Here's how the part is built. I have some questions about the finished solid (model axes, mm). Face numbers are marked on the shaded views. A direction names the side the tool comes from. Coordinates: 2 decimals unless noted, no trailing zeros. Loops run counter-clockwise (first coordinate to the right, second up) from the corner with the lowest first, then second, coordinate; pieces in that order, holes last. Notation, with made-up numbers: (74, -17) -> (122, -17) arc R7 ccw to (122, -7) -> close; hole circle Ø4 at (70, 32.25). An arc over 180 degrees is marked (long way). Answer as a JSON object with one key per item and string values. Group by question number.
1) I want a section at B-B (y = 5). Write out the boundary of the cut face in (x, z), then the cut area to 3 significant figures.
2) I want a section at C-C (z = 67.5). Write out the boundary of the cut face in (x, y), then the cut area to 3 significant figures.
3) I want a section at A-A (x = -34.5). Write out the boundary of the cut face in (y, z).
4) I'm going to push flat-ended pins straight in: pin 1 (2 mm diameter, centred on y = 11, z = 23.5, fed in from -X); pin 2 (3.5 mm diameter, centred on x = -56.5, z = 25.5, fed in from +Y); pin 3 (1 mm diameter, centred on x = -27, z = 50.5, fed in from -Y); pin 4 (4 mm diameter, centred on y = 9.5, z = 72.5, fed in from +X). Where does each tip first touch, or does it pass through?
5) I need wall thicknesses on probe 1 along X at (y, z) = (13, 14); probe 2 along Z at (x, y) = (-77, 33); probe 3 along X at (y, z) = (12, 80.5). Which ranges of each line are inside material? Lowest first, please. Write a range as [from, to].
6) Which directions (+Z, -Z, +X, -X, +Y, -Y) give clear straight access to the entire face, cutting with the end or side of a thin tool? Please do the marked faces 4, 5 and 6.
7) I want a section at D-D (x = -10.16). Count the separate pieces of the cut face and the enclosed holes in it, then the cut area to 3 significant figures.
8) If we mould it in two halves opening along Y, with no side actions, what happens to the marked faces 1, 2 and 3? For each: +Y half, -Y half, draft (parallel to the pull), parting line (faces both ways), or undercut.
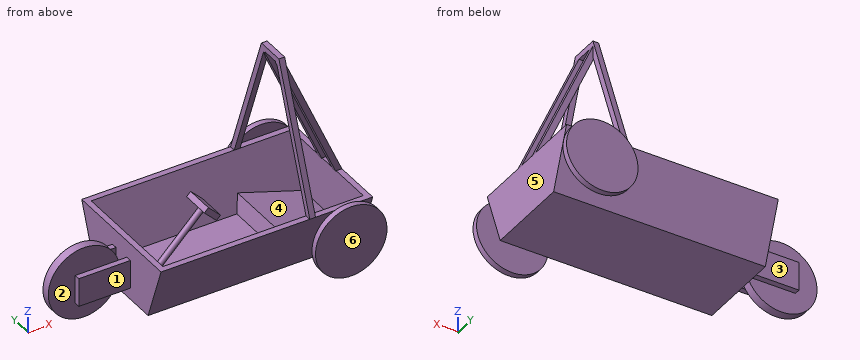
```python
from build123d import *

# Parameters (mm, degrees)
SKETCH1_W                        = 88.9
SKETCH1_H                        = 38.1
BOSS_EXTRUDE1_DEPTH              = 2.54
BOSS_EXTRUDE2_DEPTH              = 88.9
BOSS_EXTRUDE3_DEPTH              = 2.54
SKETCH5_R                        = 2.54
BOSS_EXTRUDE4_DEPTH              = 2.54
BOSS_EXTRUDE4_DIRECTION_2_REACH  = 110.401
SKETCH6_R                        = 15.875
BOSS_EXTRUDE5_DEPTH              = 2.54
BOSS_EXTRUDE6_DEPTH              = 2.54
SKETCH8_W                        = 12.7
SKETCH8_H                        = 2.54
BOSS_EXTRUDE7_DEPTH              = 22.86
SKETCH9_R                        = 2.54
BOSS_EXTRUDE8_DEPTH              = 12.7
SKETCH11_R                       = 15.875
BOSS_EXTRUDE9_DEPTH              = 1.905
BOSS_EXTRUDE9_DEPTH_BACK         = 1.905
SKETCH13_W                       = 2.54
SKETCH13_H                       = 2.53363156
BOSS_EXTRUDE10_DEPTH             = 63.5
BOSS_EXTRUDE10_DIRECTION_2_REACH = 140.326
SKETCH16_W                       = 2.54
SKETCH16_H                       = 2.54
BOSS_EXTRUDE12_DEPTH             = 63.5
BOSS_EXTRUDE12_DIRECTION_2_REACH = 150.26
BOSS_EXTRUDE14_START             = -6.254388
SKETCH18_W                       = 2.54
SKETCH18_H                       = 2.54
BOSS_EXTRUDE14_DEPTH             = 12.514761
SKETCH19_W                       = 65.643872796
SKETCH19_H                       = 2.54
BOSS_EXTRUDE15_DEPTH             = 2.54
SKETCH20_W                       = 5.651471939
SKETCH20_H                       = 13.55717745
CUT_EXTRUDE1_DEPTH               = 2.54
SKETCH21_R                       = 1.27
BOSS_EXTRUDE16_DEPTH             = 39.116
SKETCH22_W                       = 9.722484857
SKETCH22_H                       = 17.213461762
CUT_EXTRUDE2_DEPTH               = 39.116
SKETCH23_W                       = 7.62
SKETCH23_H                       = 12.7
BOSS_EXTRUDE17_DEPTH             = 2.54
BOSS_EXTRUDE18_REACH             = 161.998
BOSS_EXTRUDE18_DIRECTION_2_REACH = 161.998


with BuildPart() as part:
    # Sketch1 → Boss-Extrude1 (new body)
    with BuildSketch(Plane.XY):
        with Locations((-44.45, 19.05)):
            Rectangle(SKETCH1_W, SKETCH1_H)
    extrude(amount=BOSS_EXTRUDE1_DEPTH)

    # Sketch2 → Boss-Extrude2 (add, through all)
    with BuildSketch(Plane.ZY.offset(88.9)):
        Polygon((0, 0), (25.4, -9.24484395), (25.4, -6.541832408), (2.54, 1.778527147), align=None)
        Polygon((0, 38.1), (25.4, 47.34484395), (25.4, 44.641832408), (2.54, 36.321472853), align=None)
    extrude(amount=-BOSS_EXTRUDE2_DEPTH)

    # Sketch3 → Boss-Extrude3 (add)
    with BuildSketch(Plane(origin=(0, 0, 0), x_dir=(0, 0, -1), z_dir=(1, 0, 0))):
        Polygon((-25.4, -9.24484395), (0, 0), (0, 38.1), (-25.4, 47.34484395), align=None)
    extrude(amount=BOSS_EXTRUDE3_DEPTH)

    # Sketch5 → Boss-Extrude4 (add)
    with BuildSketch(Plane(origin=(0, 47.34484395, 0), x_dir=(-1, 0, 0), z_dir=(0, 1, 0))):
        with Locations(Location((10.16, 12.7, 0), (0, 0, 90))):
            Circle(SKETCH5_R)
    boss_extrude4 = extrude(amount=BOSS_EXTRUDE4_DEPTH)

    # Sketch5 → Boss-Extrude4 direction 2 (add, up to next)
    with BuildSketch(Plane(origin=(0, 47.34484395, 0), x_dir=(-1, 0, 0), z_dir=(0, 1, 0)), mode=Mode.PRIVATE) as boss_extrude4_direction_2_sk1:
        with Locations(Location((10.16, 12.7, 0), (0, 0, 90))):
            Circle(SKETCH5_R)
    boss_extrude4_direction_2_tool1 = extrude(boss_extrude4_direction_2_sk1.sketch, amount=-BOSS_EXTRUDE4_DIRECTION_2_REACH, mode=Mode.PRIVATE) - part.part
    boss_extrude4_direction_2 = boss_extrude4_direction_2_tool1.solids().sort_by_distance((-10.16, 47.344844, 12.7))[0]
    add(boss_extrude4_direction_2)

    # Sketch6 → Boss-Extrude5 (add)
    with BuildSketch(Plane(origin=(0, 49.88484395, 0), x_dir=(1, 0, 0), z_dir=(0, 1, 0))):
        with Locations(Location((-10.16, -12.7, 0), (0, 0, 270))):
            Circle(SKETCH6_R)
    boss_extrude5 = extrude(amount=BOSS_EXTRUDE5_DEPTH)

    # Sketch7 → Boss-Extrude6 (add)
    with BuildSketch(Plane.ZY.offset(88.9)):
        Polygon((25.4, 47.34484395), (25.4, 19.05), (0, 19.05), (0, 38.1), align=None)
    boss_extrude6 = extrude(amount=BOSS_EXTRUDE6_DEPTH)

    # Mirror1: Boss-Extrude4, Boss-Extrude4 direction 2, Boss-Extrude5, Boss-Extrude6 across plane
    add(boss_extrude4.mirror(Plane(origin=(0, 19.05, 0), x_dir=(0, 0, 1), z_dir=(0, -1, 0))))
    add(boss_extrude4_direction_2.mirror(Plane(origin=(0, 19.05, 0), x_dir=(0, 0, 1), z_dir=(0, -1, 0))))
    add(boss_extrude5.mirror(Plane(origin=(0, 19.05, 0), x_dir=(0, 0, 1), z_dir=(0, -1, 0))))
    add(boss_extrude6.mirror(Plane(origin=(0, 19.05, 0), x_dir=(0, 0, 1), z_dir=(0, -1, 0))))

    # Sketch8 → Boss-Extrude7 (add)
    with BuildSketch(Plane.ZY.offset(91.44)):
        with Locations((11.43, 24.13)):
            Rectangle(SKETCH8_W, SKETCH8_H)
        with Locations((11.43, 13.97)):
            Rectangle(SKETCH8_W, SKETCH8_H)
    extrude(amount=BOSS_EXTRUDE7_DEPTH)

    # Sketch9 → Boss-Extrude8 (add)
    with BuildSketch(Plane(origin=(0, 12.7, 0), x_dir=(-1, 0, 0), z_dir=(0, -1, 0))):
        with Locations(Location((109.22, -11.699801303, 0), (0, 0, 90))):
            Circle(SKETCH9_R)
    extrude(amount=-BOSS_EXTRUDE8_DEPTH)

    # Sketch11 → Boss-Extrude9 (add, two sides)
    with BuildSketch(Plane(origin=(0, 19.05, 0), x_dir=(-1, 0, 0), z_dir=(0, -1, 0))) as boss_extrude9_sk:
        with Locations(Location((109.22, -11.699801303, 0), (0, 0, 180))):
            Circle(SKETCH11_R)
    extrude(amount=BOSS_EXTRUDE9_DEPTH)
    extrude(boss_extrude9_sk.sketch, amount=-BOSS_EXTRUDE9_DEPTH_BACK)


with BuildPart() as body_2:
    # Sketch13 → Boss-Extrude10 (new body)
    with BuildSketch(Plane(origin=(0, -2.941300262, 8.081156055), x_dir=(-1, 0, 0), z_dir=(0, 0.34202014332566333, -0.9396926207859104))):
        with Locations((24.13, 51.903727913)):
            Rectangle(SKETCH13_W, SKETCH13_H)
    extrude(amount=-BOSS_EXTRUDE10_DEPTH)


    # Sketch13 → Boss-Extrude10 direction 2 (add, up to next)
    with BuildSketch(Plane(origin=(0, -2.941300262, 8.081156055), x_dir=(-1, 0, 0), z_dir=(0, 0.34202014332566333, -0.9396926207859104)), mode=Mode.PRIVATE) as boss_extrude10_direction_2_sk1:
        with Locations((24.13, 51.903727913)):
            Rectangle(SKETCH13_W, SKETCH13_H)
    boss_extrude10_direction_2_tool1 = extrude(boss_extrude10_direction_2_sk1.sketch, amount=BOSS_EXTRUDE10_DIRECTION_2_REACH, mode=Mode.PRIVATE) - part.part
    add(boss_extrude10_direction_2_tool1.solids().sort_by_distance((-24.13, 45.83225, 25.833277))[0])


with BuildPart() as boss_extrude12_tool:
    # Sketch16 → Boss-Extrude12 (new body)
    with BuildSketch(Plane(origin=(0, 7.398153621, 20.326260019), x_dir=(-1, 0, 0), z_dir=(0, 0.34202014332566943, 0.9396926207859081))):
        with Locations((24.13, 16.104623281)):
            Rectangle(SKETCH16_W, SKETCH16_H)
    extrude(amount=BOSS_EXTRUDE12_DEPTH)


with BuildPart() as part_1:
    add(part.part)


with BuildPart() as part_2:
    # Boss-Extrude12: joined with boss_extrude12_tool
    add(part_1.part.fuse(boss_extrude12_tool.part, tol=0.00001))

    # Sketch16 → Boss-Extrude12 direction 2 (add, up to next)
    with BuildSketch(Plane(origin=(0, 7.398153621, 20.326260019), x_dir=(-1, 0, 0), z_dir=(0, 0.34202014332566943, 0.9396926207859081)), mode=Mode.PRIVATE) as boss_extrude12_direction_2_sk1:
        with Locations((24.13, 16.104623281)):
            Rectangle(SKETCH16_W, SKETCH16_H)
    boss_extrude12_direction_2_tool1 = extrude(boss_extrude12_direction_2_sk1.sketch, amount=-BOSS_EXTRUDE12_DIRECTION_2_REACH, mode=Mode.PRIVATE) - part_2.part
    add(boss_extrude12_direction_2_tool1.solids().sort_by_distance((-24.13, -7.735242, 25.834366))[0])


    add(body_2.part)  # Boss-Extrude14 merges body 2
    # Sketch18 → Boss-Extrude14 (add)
    with BuildSketch(Plane(origin=(0, 19.05, 0), x_dir=(-1, 0, 0), z_dir=(0, -1, 0)).offset(BOSS_EXTRUDE14_START)):
        with Locations((24.13, -84.669212584)):
            Rectangle(SKETCH18_W, SKETCH18_H)
    extrude(amount=BOSS_EXTRUDE14_DEPTH)

    # Sketch19 → Boss-Extrude15 (add)
    with BuildSketch(Plane(origin=(11.464782442, 0, 5.020852199), x_dir=(-0.40115477823907125, 0, 0.9160102859116602), z_dir=(-0.9160102859116602, 0, -0.40115477823907125))):
        with Locations((55.069664523, 14.059627436)):
            Rectangle(SKETCH19_W, SKETCH19_H)
        with Locations((55.069664523, 24.033595411)):
            Rectangle(SKETCH19_W, SKETCH19_H)
    extrude(amount=BOSS_EXTRUDE15_DEPTH)

    # Sketch20 → Cut-Extrude1 (cut)
    with BuildSketch(Plane.ZY.offset(25.4)):
        with Locations((83.113476615, 18.525006686)):
            Rectangle(SKETCH20_W, SKETCH20_H)
    extrude(amount=CUT_EXTRUDE1_DEPTH, mode=Mode.SUBTRACT)

    # Sketch21 → Boss-Extrude16 (add)
    with BuildSketch(Plane(origin=(-43.18, 0, -43.18), x_dir=(0, -1, 0), z_dir=(0.7071067811865488, 0, 0.7071067811865464))):
        with Locations(Location((-19.05, -57.037844072, 0), (0, 0, 270))):
            Circle(SKETCH21_R)
    extrude(amount=BOSS_EXTRUDE16_DEPTH)

    # Sketch22 → Cut-Extrude2 (cut)
    with BuildSketch(Plane(origin=(0, 0, 0), x_dir=(-1, 0, 0), z_dir=(0, 0, -1))):
        with Locations((79.946093386, 21.082088855)):
            Rectangle(SKETCH22_W, SKETCH22_H)
    extrude(amount=CUT_EXTRUDE2_DEPTH, mode=Mode.SUBTRACT)

    # Sketch23 → Boss-Extrude17 (add)
    with BuildSketch(Plane(origin=(-15.520811147, 0, -15.520811147), x_dir=(0.7071067811865465, 0, -0.7071067811865487), z_dir=(0.7071067811865487, 0, 0.7071067811865465))):
        with Locations((-57.037844072, 19.05)):
            Rectangle(SKETCH23_W, SKETCH23_H)
    extrude(amount=BOSS_EXTRUDE17_DEPTH)

    # Sketch25 → Boss-Extrude18 (add, up to next)
    with BuildSketch(Plane(origin=(0, 36.321472853, 0), x_dir=(-1, 0, 0), z_dir=(0, 1, 0)), mode=Mode.PRIVATE) as boss_extrude18_sk1:
        Polygon((0, 2.54), (27.469218062, 9.900354796), (29.441419185, 2.54), align=None)
    boss_extrude18_tool1 = extrude(boss_extrude18_sk1.sketch, amount=-BOSS_EXTRUDE18_REACH, mode=Mode.PRIVATE) - part_2.part
    add(boss_extrude18_tool1.solids().sort_by_distance((-18.970212, 36.321473, 4.993452))[0])

    # Sketch25 → Boss-Extrude18 direction 2 (add, up to next)
    with BuildSketch(Plane(origin=(0, 36.321472853, 0), x_dir=(-1, 0, 0), z_dir=(0, 1, 0)), mode=Mode.PRIVATE) as boss_extrude18_direction_2_sk1:
        Polygon((0, 2.54), (27.469218062, 9.900354796), (29.441419185, 2.54), align=None)
    boss_extrude18_direction_2_tool1 = extrude(boss_extrude18_direction_2_sk1.sketch, amount=BOSS_EXTRUDE18_DIRECTION_2_REACH, mode=Mode.PRIVATE) - part_2.part
    add(boss_extrude18_direction_2_tool1.solids().sort_by_distance((-18.970212, 36.321473, 4.993452))[0])


solid = part_2.part
```
Determined:
{
 "1": {"outline": "(-91.44, 0) -> (2.54, 0) -> (2.54, 25.4) -> (0, 25.4) -> (0, 2.54) -> (-27.47, 9.9) -> (-29.44, 2.54) -> (-88.9, 2.54) -> (-88.9, 25.4) -> (-91.44, 25.4) -> close; (-25.4, 57.11) -> (-22.86, 57.11) -> (-22.86, 64.54) -> (-25.4, 64.54) -> close", "area": "482 mm^2"},
 "2": {"outline": "(-25.4, 6.08) -> (-22.86, 6.08) -> (-22.86, 8.78) -> (-25.4, 8.78) -> close; (-25.4, 29.32) -> (-22.86, 29.32) -> (-22.86, 32.01) -> (-25.4, 32.01) -> close; (-18.67, 12.79) -> (-15.9, 12.79) -> (-15.9, 15.33) -> (-18.67, 15.33) -> close; (-18.67, 22.76) -> (-15.9, 22.76) -> (-15.9, 25.3) -> (-18.67, 25.3) -> close", "area": "27.8 mm^2"},
 "3": {"outline": "(-9.24, 25.4) -> (0, 0) -> (38.1, 0) -> (47.34, 25.4) -> (44.64, 25.4) -> (36.32, 2.54) -> (1.78, 2.54) -> (-6.54, 25.4) -> close"},
 "4": {"pin 1": "x = -91.44", "pin 2": "y = 47.34", "pin 3": "through", "pin 4": "x = -22.86"},
 "5": {"probe 1": "[-114.3, -88.9], [0, 2.54]", "probe 2": "[0, 2.54]", "probe 3": "[-25.4, -22.86]"},
 "6": {"face 4": "none", "face 5": "+Z, -Z, +X", "face 6": "+Z, -Z, +X, -X, -Y"},
 "7": {"separate pieces": "3", "enclosed holes": "0", "area": "586 mm^2"},
 "8": {"face 1": "-Y half", "face 2": "undercut", "face 3": "+Y half"}
}
